Here's how the part is built. I have some questions about the finished solid (model axes, mm). Coordinates: 2 decimals unless noted, no trailing zeros. Write each loop counter-clockwise with the first axis right and the second up, starting at its lowest first coordinate (ties: lowest second). Pieces come first, ordered by that corner, then holes. Notation, with made-up numbers: (-10, -39.75) -> (19, -39.75) arc R20 ccw to (19, -3.75) -> close; hole circle Ø3 at (33, -35). An arc over 180 degrees is marked (long way). Use a Markdown table: item, result. Add a question column.
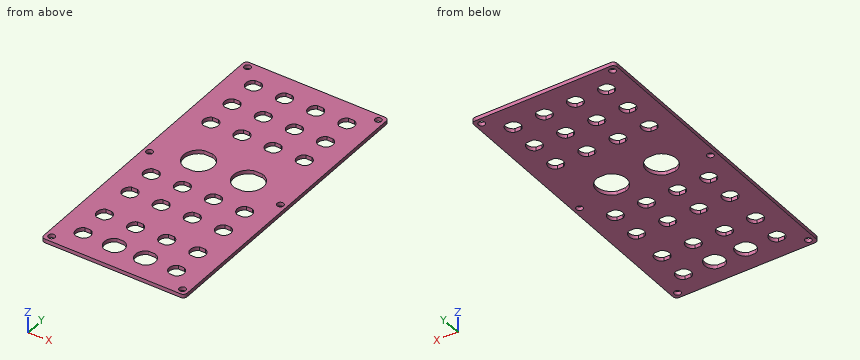
```python
from build123d import *

# Parameters (mm, degrees)
SKETCH1_W            = 115
SKETCH1_H            = 240
BOSS_EXTRUDE1_DEPTH  = 3
CUT_EXTRUDE1_DEPTH   = 3
LPATTERN1_COUNT      = 4
LPATTERN1_PITCH      = 25
LPATTERN1_COUNT_DIR2 = 2
LPATTERN1_PITCH_DIR2 = 25
CUT_EXTRUDE2_DEPTH   = 3
LPATTERN2_COUNT      = 4
LPATTERN2_PITCH      = 25
LPATTERN2_COUNT_DIR2 = 3
LPATTERN2_PITCH_DIR2 = 25
CUT_EXTRUDE3_DEPTH   = 3
CUT_EXTRUDE4_DEPTH   = 3
LPATTERN3_COUNT      = 4
LPATTERN3_PITCH      = 25
LPATTERN3_COUNT_DIR2 = 2
LPATTERN3_PITCH_DIR2 = 25
CUT_EXTRUDE5_DEPTH   = 3
M5_CLEARANCE_HOLE1_D = 5.3
FILLET1_R            = 3


with BuildPart() as part:
    # Sketch1 → Boss-Extrude1 (new body)
    with BuildSketch(Plane.XY):
        with Locations((57.5, 120)):
            Rectangle(SKETCH1_W, SKETCH1_H)
    extrude(amount=BOSS_EXTRUDE1_DEPTH)

    # Sketch2 → Cut-Extrude1 (cut)
    with BuildSketch(Plane.XY.offset(3)):
        with BuildLine():
            Line((22.397915762, 25.5), (17.602084238, 25.5))
            ThreePointArc((17.602084238, 25.5), (14, 20), (17.602084238, 14.5))
            Line((17.602084238, 14.5), (22.397915762, 14.5))
            ThreePointArc((22.397915762, 14.5), (26, 20), (22.397915762, 25.5))
        make_face()
    cut_extrude1 = extrude(amount=-CUT_EXTRUDE1_DEPTH, mode=Mode.SUBTRACT)

    # LPattern1: Cut-Extrude1 4 × 2, 2 skipped
    with Locations(*[(i * LPATTERN1_PITCH, j * LPATTERN1_PITCH_DIR2, 0) for i in range(LPATTERN1_COUNT) for j in range(LPATTERN1_COUNT_DIR2) if (i, j) not in ((0, 0), (1, 0), (2, 0))]):
        add(cut_extrude1, mode=Mode.SUBTRACT)

    # Sketch3 → Cut-Extrude2 (cut)
    with BuildSketch(Plane.XY.offset(3)):
        with BuildLine():
            Line((22.397915762, 214.5), (17.602084238, 214.5))
            ThreePointArc((17.602084238, 214.5), (14, 220), (17.602084238, 225.5))
            Line((17.602084238, 225.5), (22.397915762, 225.5))
            ThreePointArc((22.397915762, 225.5), (26, 220), (22.397915762, 214.5))
        make_face()
    cut_extrude2 = extrude(amount=-CUT_EXTRUDE2_DEPTH, mode=Mode.SUBTRACT)

    # LPattern2: Cut-Extrude2 4 × 3
    with Locations(*[(i * LPATTERN2_PITCH, -j * LPATTERN2_PITCH_DIR2, 0) for i in range(LPATTERN2_COUNT) for j in range(LPATTERN2_COUNT_DIR2) if (i, j) != (0, 0)]):
        add(cut_extrude2, mode=Mode.SUBTRACT)

    # Sketch4 → Cut-Extrude3 (cut)
    with BuildSketch(Plane.XY.offset(3)):
        with BuildLine():
            Line((42.216117819, 27.5), (47.783882181, 27.5))
            ThreePointArc((47.783882181, 27.5), (53, 20), (47.783882181, 12.5))
            Line((47.783882181, 12.5), (42.216117819, 12.5))
            ThreePointArc((42.216117819, 12.5), (37, 20), (42.216117819, 27.5))
        make_face()
    cut_extrude3 = extrude(amount=-CUT_EXTRUDE3_DEPTH, mode=Mode.SUBTRACT)

    # Mirror2: Cut-Extrude3 across plane
    add(cut_extrude3.mirror(Plane.ZY.offset(-57.5)), mode=Mode.SUBTRACT)

    # Sketch5 → Cut-Extrude4 (cut)
    with BuildSketch(Plane.XY.offset(3)):
        with BuildLine():
            Line((22.397915762, 80.5), (17.602084238, 80.5))
            ThreePointArc((17.602084238, 80.5), (14, 75), (17.602084238, 69.5))
            Line((17.602084238, 69.5), (22.397915762, 69.5))
            ThreePointArc((22.397915762, 69.5), (26, 75), (22.397915762, 80.5))
        make_face()
    cut_extrude4 = extrude(amount=-CUT_EXTRUDE4_DEPTH, mode=Mode.SUBTRACT)

    # LPattern3: Cut-Extrude4 4 × 2
    with Locations(*[(i * LPATTERN3_PITCH, j * LPATTERN3_PITCH_DIR2, 0) for i in range(LPATTERN3_COUNT) for j in range(LPATTERN3_COUNT_DIR2) if (i, j) != (0, 0)]):
        add(cut_extrude4, mode=Mode.SUBTRACT)

    # Sketch7 → Cut-Extrude5 (cut)
    with BuildSketch(Plane.XY.offset(3)):
        with BuildLine():
            Line((34.0721727, 141.5), (40.9278273, 141.5))
            ThreePointArc((40.9278273, 141.5), (49.5, 130), (40.9278273, 118.5))
            Line((40.9278273, 118.5), (34.0721727, 118.5))
            ThreePointArc((34.0721727, 118.5), (25.5, 130), (34.0721727, 141.5))
        make_face()
    cut_extrude5 = extrude(amount=-CUT_EXTRUDE5_DEPTH, mode=Mode.SUBTRACT)

    # Mirror3: Cut-Extrude5 across plane
    add(cut_extrude5.mirror(Plane.ZY.offset(-57.5)), mode=Mode.SUBTRACT)

    # M5 Clearance Hole1 (through all)
    with Locations(Plane.XY.offset(3)):
        with Locations((5, 235), (5, 5), (110, 5), (110, 235), (5, 120), (110, 120)):
            Hole(M5_CLEARANCE_HOLE1_D / 2)

    # Fillet1
    fillet1_edges = [part.edges().sort_by_distance(p)[0] for p in [
        (0, 240, 1.5),
        (115, 240, 1.5),
        (115, 0, 1.5),
        (0, 0, 1.5),
    ]]
    fillet(fillet1_edges, radius=FILLET1_R)


solid = part.part
```
Q1. Please list where these lines run through material, in increasing order: line 1 (Y direction, x = 110, z = 0.9); line 2 (Y direction, x = 81, z = 0.9); line 3 (X direction, y = 43, z = 0.95).
Q2. Suppose I cut it at B-B, the plane z = 2.25. State how many separate pieces and enclosed holes the cut face has, and give its area (3 significant figures).
Q3. Suppose I cut it at C-C, the plane y = 74. Write out the boundary of the cut face in (x, z), and give its area (3 significant figures).
Q4. Suppose I cut it at A-A, the plane y = 18.5. Write out the boundary of the cut face in (x, z).
Answer key:
| question | item | result |
|---|---|---|
| 1 | line 1 | y = 0 to 2.35, 7.65 to 117.35, 122.65 to 232.35, 237.65 to 240 |
| 1 | line 2 | y = 0 to 118.52, 141.48 to 240 |
| 1 | line 3 | x = 0 to 14.34, 25.66 to 39.34, 50.66 to 64.34, 75.66 to 89.34, 100.66 to 115 |
| 2 | separate pieces | 1 |
| 2 | enclosed holes | 36 |
| 2 | area | 23,300 mm^2 |
| 3 | outline | (0, 0) -> (14.08, 0) -> (14.08, 3) -> (0, 3) -> close; (25.92, 0) -> (39.08, 0) -> (39.08, 3) -> (25.92, 3) -> close; (50.92, 0) -> (64.08, 0) -> (64.08, 3) -> (50.92, 3) -> close; (75.92, 0) -> (89.08, 0) -> (89.08, 3) -> (75.92, 3) -> close; (100.92, 0) -> (115, 0) -> (115, 3) -> (100.92, 3) -> close |
| 3 | area | 203 mm^2 |
| 4 | outline | (0, 0) -> (14.19, 0) -> (14.19, 3) -> (0, 3) -> close; (25.81, 0) -> (37.14, 0) -> (37.14, 3) -> (25.81, 3) -> close; (52.86, 0) -> (62.14, 0) -> (62.14, 3) -> (52.86, 3) -> close; (77.86, 0) -> (89.19, 0) -> (89.19, 3) -> (77.86, 3) -> close; (100.81, 0) -> (115, 0) -> (115, 3) -> (100.81, 3) -> close |
